from build123d import *

# Parameters (mm, degrees)
ESQUISSE1_W                         = 180
ESQUISSE1_H                         = 80
BOSS_EXTRU_1_DEPTH                  = 4
ENL_V_MAT_EXTRU_1_DEPTH             = 4
ENL_V_MAT_EXTRU_2_DEPTH             = 4
ENL_V_MAT_EXTRU_5_REACH             = 6
ESQUISSE11_W                        = 12
ESQUISSE11_H                        = 60
ENL_V_MAT_EXTRU_5_DIRECTION_2_DEPTH = 1
ENL_V_MAT_EXTRU_6_REACH             = 6
ESQUISSE14_R                        = 7.5


with BuildPart() as part:
    # Esquisse1 → Boss.-Extru.1 (new body)
    with BuildSketch(Plane(origin=(0, 0, 0), x_dir=(1, 0, 0), z_dir=(0, 1, 0))):
        with Locations((90, 40)):
            Rectangle(ESQUISSE1_W, ESQUISSE1_H)
    extrude(amount=BOSS_EXTRU_1_DEPTH)

    # Esquisse2 → Enlèv. mat.-Extru.1 (cut)
    with BuildSketch(Plane(origin=(0, 4, 0), x_dir=(1, 0, 0), z_dir=(0, 1, 0))):
        Polygon((30, 0), (0, 15), (0, 0), align=None)
        Polygon((30, 80), (0, 65), (0, 80), align=None)
        Polygon((150, 0), (180, 15), (180, 0), align=None)
        Polygon((150, 80), (180, 80), (180, 65), align=None)
    extrude(amount=-ENL_V_MAT_EXTRU_1_DEPTH, mode=Mode.SUBTRACT)

    # Esquisse3 → Enlèv. mat.-Extru.2 (cut)
    with BuildSketch(Plane(origin=(0, 4, 0), x_dir=(1, 0, 0), z_dir=(0, 1, 0))):
        with BuildLine():
            Line((65.05, 38), (65.05, 18))
            ThreePointArc((65.05, 18), (64, 16.95), (62.95, 18))
            Line((62.95, 18), (62.95, 38))
            ThreePointArc((62.95, 38), (64, 39.05), (65.05, 38))
        make_face()
        with BuildLine():
            Line((50.95, 18), (50.95, 38))
            ThreePointArc((50.95, 38), (52, 39.05), (53.05, 38))
            Line((53.05, 38), (53.05, 18))
            ThreePointArc((53.05, 18), (52, 16.95), (50.95, 18))
        make_face()
        with BuildLine():
            Line((129.05, 18), (129.05, 38))
            ThreePointArc((129.05, 38), (128, 39.05), (126.95, 38))
            Line((126.95, 38), (126.95, 18))
            ThreePointArc((126.95, 18), (128, 16.95), (129.05, 18))
        make_face()
        with BuildLine():
            Line((114.95, 38), (114.95, 18))
            ThreePointArc((114.95, 18), (116, 16.95), (117.05, 18))
            Line((117.05, 18), (117.05, 38))
            ThreePointArc((117.05, 38), (116, 39.05), (114.95, 38))
        make_face()
        with BuildLine():
            Line((50.95, 62), (50.95, 42))
            ThreePointArc((50.95, 42), (52, 40.95), (53.05, 42))
            Line((53.05, 42), (53.05, 62))
            ThreePointArc((53.05, 62), (52, 63.05), (50.95, 62))
        make_face()
        with BuildLine():
            Line((65.05, 42), (65.05, 62))
            ThreePointArc((65.05, 62), (64, 63.05), (62.95, 62))
            Line((62.95, 62), (62.95, 42))
            ThreePointArc((62.95, 42), (64, 40.95), (65.05, 42))
        make_face()
        with BuildLine():
            Line((114.95, 42), (114.95, 62))
            ThreePointArc((114.95, 62), (116, 63.05), (117.05, 62))
            Line((117.05, 62), (117.05, 42))
            ThreePointArc((117.05, 42), (116, 40.95), (114.95, 42))
        make_face()
        with BuildLine():
            Line((129.05, 62), (129.05, 42))
            ThreePointArc((129.05, 42), (128, 40.95), (126.95, 42))
            Line((126.95, 42), (126.95, 62))
            ThreePointArc((126.95, 62), (128, 63.05), (129.05, 62))
        make_face()
    extrude(amount=-ENL_V_MAT_EXTRU_2_DEPTH, mode=Mode.SUBTRACT)

    # Esquisse11 → Enlèv. mat.-Extru.5 (cut, up to next)
    with BuildSketch(Plane(origin=(0, 4, 0), x_dir=(1, 0, 0), z_dir=(0, 1, 0)), mode=Mode.PRIVATE) as enl_v_mat_extru_5_sk1:
        with Locations((34, 40)):
            Rectangle(ESQUISSE11_W, ESQUISSE11_H)
    enl_v_mat_extru_5_tool1 = extrude(enl_v_mat_extru_5_sk1.sketch, amount=-ENL_V_MAT_EXTRU_5_REACH, mode=Mode.PRIVATE) & part.part
    add(enl_v_mat_extru_5_tool1.solids().sort_by_distance((34, 4, -40))[0], mode=Mode.SUBTRACT)
    # Esquisse11 → Enlèv. mat.-Extru.5 (cut, up to next)
    with BuildSketch(Plane(origin=(0, 4, 0), x_dir=(1, 0, 0), z_dir=(0, 1, 0)), mode=Mode.PRIVATE) as enl_v_mat_extru_5_sk2:
        with Locations((146, 40)):
            Rectangle(ESQUISSE11_W, ESQUISSE11_H)
    enl_v_mat_extru_5_tool2 = extrude(enl_v_mat_extru_5_sk2.sketch, amount=-ENL_V_MAT_EXTRU_5_REACH, mode=Mode.PRIVATE) & part.part
    add(enl_v_mat_extru_5_tool2.solids().sort_by_distance((146, 4, -40))[0], mode=Mode.SUBTRACT)

    # Esquisse11 → Enlèv. mat.-Extru.5 direction 2 (cut)
    with BuildSketch(Plane(origin=(0, 4, 0), x_dir=(1, 0, 0), z_dir=(0, 1, 0))):
        with Locations((34, 40)):
            Rectangle(ESQUISSE11_W, ESQUISSE11_H)
        with Locations((146, 40)):
            Rectangle(ESQUISSE11_W, ESQUISSE11_H)
    extrude(amount=ENL_V_MAT_EXTRU_5_DIRECTION_2_DEPTH, mode=Mode.SUBTRACT)

    # Esquisse14 → Enlèv. mat.-Extru.6 (cut, up to next)
    with BuildSketch(Plane(origin=(0, 4, 0), x_dir=(1, 0, 0), z_dir=(0, 1, 0)), mode=Mode.PRIVATE) as enl_v_mat_extru_6_sk1:
        with Locations((90, 60)):
            Circle(ESQUISSE14_R)
    enl_v_mat_extru_6_tool1 = extrude(enl_v_mat_extru_6_sk1.sketch, amount=-ENL_V_MAT_EXTRU_6_REACH, mode=Mode.PRIVATE) & part.part
    add(enl_v_mat_extru_6_tool1.solids().sort_by_distance((90, 4, -60))[0], mode=Mode.SUBTRACT)
    # Esquisse14 → Enlèv. mat.-Extru.6 (cut, up to next)
    with BuildSketch(Plane(origin=(0, 4, 0), x_dir=(1, 0, 0), z_dir=(0, 1, 0)), mode=Mode.PRIVATE) as enl_v_mat_extru_6_sk2:
        with Locations((90, 40)):
            Circle(ESQUISSE14_R)
    enl_v_mat_extru_6_tool2 = extrude(enl_v_mat_extru_6_sk2.sketch, amount=-ENL_V_MAT_EXTRU_6_REACH, mode=Mode.PRIVATE) & part.part
    add(enl_v_mat_extru_6_tool2.solids().sort_by_distance((90, 4, -40))[0], mode=Mode.SUBTRACT)
    # Esquisse14 → Enlèv. mat.-Extru.6 (cut, up to next)
    with BuildSketch(Plane(origin=(0, 4, 0), x_dir=(1, 0, 0), z_dir=(0, 1, 0)), mode=Mode.PRIVATE) as enl_v_mat_extru_6_sk3:
        with Locations((90, 20)):
            Circle(ESQUISSE14_R)
    enl_v_mat_extru_6_tool3 = extrude(enl_v_mat_extru_6_sk3.sketch, amount=-ENL_V_MAT_EXTRU_6_REACH, mode=Mode.PRIVATE) & part.part
    add(enl_v_mat_extru_6_tool3.solids().sort_by_distance((90, 4, -20))[0], mode=Mode.SUBTRACT)


solid = part.part
Part model, mm, in its own coordinate system. A direction names the side the tool comes from. Round coordinates to 2 decimals unless told otherwise and drop trailing zeros. Order: outer loops, then holes, each group sorted by start corner. A loop starts at its lowest first (then second) coordinate and runs counter-clockwise, first axis right, second up. Notation, with made-up numbers: (-18, 80.5) -> (-3, 80.5) arc R21 ccw to (-3, 88.5) -> close; hole circle Ø1 at (53, 40.5). An arc over 180 degrees is marked (long way). Put each result on its own line as item: value.
Q1. Pull direction X, two halves, no side cores. Call faces 1 (the face through (165.2, 2, -72.4)), 2 (the face through (146, 2, -10)), 3 (the face through (15.2, 2, -72.6)): pulls with the +X half, pulls with the -X half, needs draft (parallel to the pull), parting line crosses it, or undercut.
From the geometry:
face 1: pulls with the +X half
face 2: undercut
face 3: pulls with the -X half
Q2. Tool access for faces 4 (the face through (164.8, 2, -7.4)), 5 (the face through (40, 2, -40)): list every direction of +Z, -Z, +X, -X, +Y, -Y with a clear straight run to the whole face (end or side of a thin tool).
From the geometry:
face 4: +Z, +X, +Y, -Y
face 5: +Y, -Y
Q3. Band-saw the part on D-D (z = -7). Give the cut face in (x, y).
From the geometry:
outline: (16, 0) -> (164, 0) -> (164, 4) -> (16, 4) -> close
Q4. Band-saw the part on C-C (x = 18.5). Give the cut face in (y, z), and give its area (3 significant figures).
From the geometry:
outline: (0, -74.25) -> (4, -74.25) -> (4, -5.75) -> (0, -5.75) -> close
area: 274 mm2
Q5. Band-saw the part on B-B (y = 1.8). State how many separate pieces and enclosed holes the cut face has, and give its area (3 significant figures).
From the geometry:
separate pieces: 1
enclosed holes: 13
area: 11,200 mm2
Q6. Wall check: line 1 (Z direction, x = 116, y = 0.8); line 2 (Z direction, x = 90, y = 1.1); line 3 (X direction, y = 0.65, z = -40). Give the ranges that are in metal, low to high. Write a range as [from, to].
From the geometry:
line 1: z = [-80, -63.05], [-40.95, -39.05], [-16.95, 0]
line 2: z = [-80, -67.5], [-52.5, -47.5], [-32.5, -27.5], [-12.5, 0]
line 3: x = [0, 28], [40, 82.5], [97.5, 140], [152, 180]
Q7. Pin check, flat tips, straight feed: pin 1 Ø9 at (x, z) = (90, -20) entering from -Y; pin 2 Ø1 at (y, z) = (2.5, -70.5) entering from +X. Stop position of each tip, or through.
From the geometry:
pin 1: passes through
pin 2: stops at x = 170
Q8. Band-saw the part on A-A (x = 90). Give the cut face in (y, z).
From the geometry:
outline: (0, -80) -> (4, -80) -> (4, -67.5) -> (0, -67.5) -> close; (0, -52.5) -> (4, -52.5) -> (4, -47.5) -> (0, -47.5) -> close; (0, -32.5) -> (4, -32.5) -> (4, -27.5) -> (0, -27.5) -> close; (0, -12.5) -> (4, -12.5) -> (4, 0) -> (0, 0) -> close
